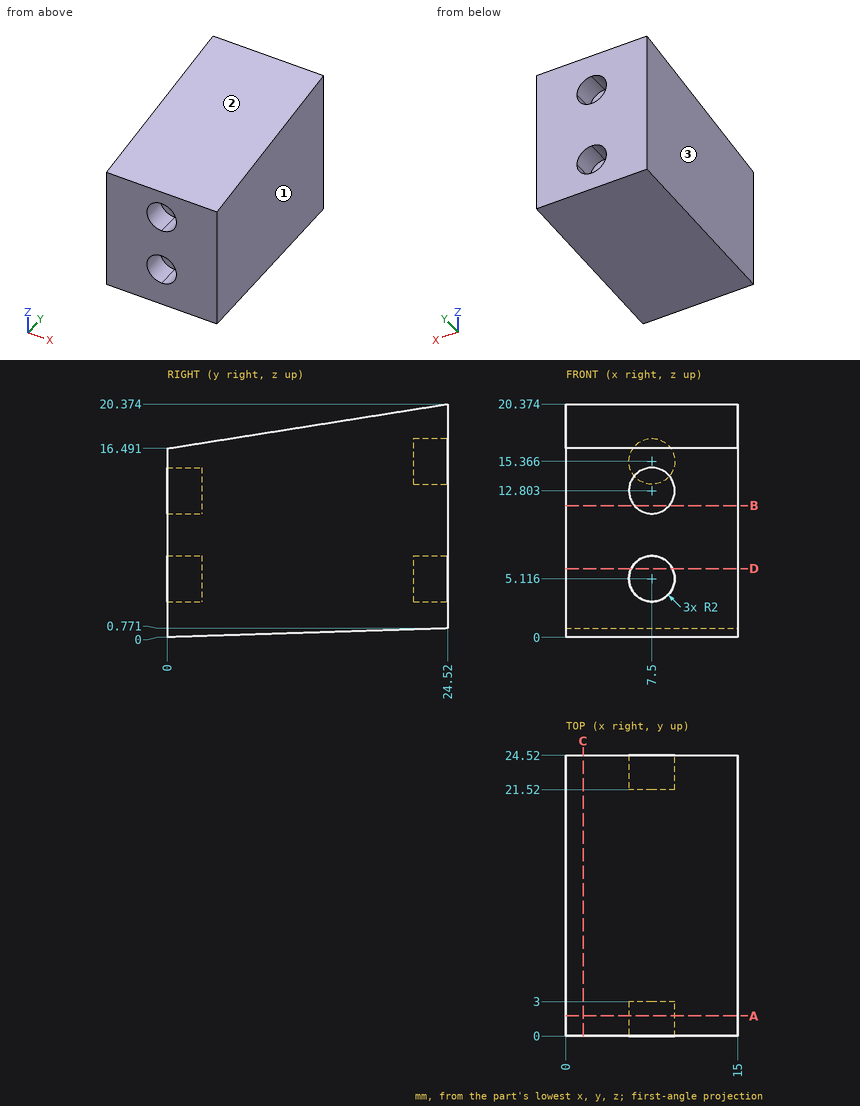
Could you check a few things on this drawing? It's one solid part, dimensions in mm from its lowest x, y, z. Round coordinates to 2 decimals unless told otherwise and drop trailing zeros. Order: outer loops, then holes, each group sorted by start corner. A loop starts at its lowest first (then second) coordinate and runs counter-clockwise, first axis right, second up.
(1) Imagine slicing it at C-C (x = 1.5). Write out the boundary of the cut face in (y, z) (1 decimal).
Response values:
outline: (0, 0) - (24.5, 0.8) - (24.5, 20.4) - (0, 16.5) - close
(2) I'm going to push flat-ended pins straight in: pin 1 (1.2 mm diameter, centred on x = 7, z = 4.5, fed in from +Y); pin 2 (5 mm diameter, centred on x = 7.5, z = 14.5, fed in from +Y); pin 3 (4 mm diameter, centred on x = 8, y = 11.5, fed in from -Z); pin 4 (6 mm diameter, centred on x = 5.5, y = 18.5, fed in from +Z). Where does each tip first touch, or does it pass through?
Response values:
pin 1: stops at y = 21.52
pin 2: stops at y = 24.52
pin 3: stops at z = 0.3
pin 4: stops at z = 19.9
(3) Imagine slicing it at D-D (z = 6). Write out the boundary of the cut face in (x, y).
Response values:
outline: (0, 0) - (5.71, 0) - (5.71, 3) - (9.29, 3) - (9.29, 0) - (15, 0) - (15, 24.52) - (9.29, 24.52) - (9.29, 21.52) - (5.71, 21.52) - (5.71, 24.52) - (0, 24.52) - close
(4) Please list where these lines run through material, in increasing order: line 1 along Z through (x, y) = (6.25, 2.75) (1 decimal); line 2 along Z through (x, y) = (7.75, 23); line 3 along Y through (x, z) = (6.5, 3.5).
Response values:
line 1: z = 0.1 to 3.6, 6.7 to 11.2, 14.4 to 16.9
line 2: z = 0.72 to 3.13, 7.1 to 13.38, 17.35 to 20.13
line 3: y = 3 to 21.52
(5) Imagine slicing it at A-A (y = 1.75). Write out the boundary of the cut face in (x, z) (1 decimal).
Response values:
outline: (0, 0.1) - (15, 0.1) - (15, 16.8) - (0, 16.8) - close; hole circle Ø4 at (7.5, 5.1); hole circle Ø4 at (7.5, 12.8)
(6) Imagine slicing it at B-B (z = 11.5). Write out the boundary of the cut face in (x, y), plus the area to 3 significant figures.
Response values:
outline: (0, 0) - (5.98, 0) - (5.98, 3) - (9.02, 3) - (9.02, 0) - (15, 0) - (15, 24.52) - (0, 24.52) - close
area: 359 mm2
(7) If we mould it in two halves opening along X, with no side actions, what happens to the marked faces 1, 2 and 3? For each: released by +X, released by -X, zero draft, split by the parting line, or undercut.
Response values:
face 1: released by +X
face 2: zero draft
face 3: released by -X
